Source: CAD feature listing. Evaluate the final solid. Frame: model axes, mm. A direction names the side the tool comes from. Round coordinates to 2 decimals unless told otherwise and drop trailing zeros. Write each loop counter-clockwise with the first axis right and the second up, starting at its lowest first coordinate (ties: lowest second). Pieces come first, ordered by that corner, then holes. Notation, with made-up numbers: (-37, -7.75) -> (-33, -7.75) arc R29 ccw to (-33, 16.25) -> close; hole circle Ø2 at (-35, 73). An arc over 180 degrees is marked (long way). Return JSON: item names as keys, results as strings. Group by question number.
from build123d import *

# Parameters (mm, degrees)
SKETCH2_R           = 13.25
SKETCH2_R_2         = 6
BOSS_EXTRUDE1_DEPTH = 5
SKETCH3_R           = 2.25
SKETCH3_R_2         = 1.25
CUT_EXTRUDE1_DEPTH  = 6


with BuildPart() as part:
    # Sketch2 → Boss-Extrude1 (new body)
    with BuildSketch(Plane.XY):
        with BuildLine():
            ThreePointArc((15.576905983, -13.25), (-20.45, 0), (15.576905983, 13.25))
            Line((15.576905983, 13.25), (25.796075283, 13.25))
            ThreePointArc((25.796075283, 13.25), (-29, 0), (25.796075283, -13.25))
            Line((25.796075283, -13.25), (15.576905983, -13.25))
        make_face()
        with BuildLine():
            ThreePointArc((20.228754287, -3), (18.621948121, -8.451363686), (15.576905983, -13.25))
            Line((15.576905983, -13.25), (25.796075283, -13.25))
            ThreePointArc((25.796075283, -13.25), (27.796785579, -8.266723138), (28.844410204, -3))
            Line((28.844410204, -3), (20.228754287, -3))
        make_face()
        with BuildLine():
            Line((25.796075283, 13.25), (15.576905983, 13.25))
            ThreePointArc((15.576905983, 13.25), (18.621948121, 8.451363686), (20.228754287, 3))
            Line((20.228754287, 3), (28.844410204, 3))
            ThreePointArc((28.844410204, 3), (27.796785579, 8.266723138), (25.796075283, 13.25))
        make_face()
        with BuildLine():
            Line((100, 13.25), (25.796075283, 13.25))
            ThreePointArc((25.796075283, 13.25), (27.796785579, 8.266723138), (28.844410204, 3))
            Line((28.844410204, 3), (50, 3))
            Line((50, 3), (80, 3))
            ThreePointArc((80, 3), (82.121320344, 2.121320344), (83, 0))
            ThreePointArc((83, 0), (82.121320344, -2.121320344), (80, -3))
            Line((80, -3), (50, -3))
            Line((50, -3), (28.844410204, -3))
            ThreePointArc((28.844410204, -3), (27.796785579, -8.266723138), (25.796075283, -13.25))
            Line((25.796075283, -13.25), (100, -13.25))
            ThreePointArc((100, -13.25), (86.75, 0), (100, 13.25))
        make_face()
        with Locations((100, 0)):
            Circle(SKETCH2_R)
        with Locations((100, 0)):
            Circle(SKETCH2_R_2, mode=Mode.SUBTRACT)
    extrude(amount=BOSS_EXTRUDE1_DEPTH)

    # Sketch3 → Cut-Extrude1 (cut, through all)
    with BuildSketch(Plane.XY.offset(5)):
        with Locations((17.67766953, 17.67766953)):
            Circle(SKETCH3_R)
        with Locations((17.67766953, -17.67766953)):
            Circle(SKETCH3_R)
        with Locations((-17.67766953, -17.67766953)):
            Circle(SKETCH3_R)
        with Locations((-17.67766953, 17.67766953)):
            Circle(SKETCH3_R)
        with Locations((100, 10.25)):
            Circle(SKETCH3_R_2)
        with Locations((108.876760389, 5.125)):
            Circle(SKETCH3_R_2)
        with Locations((91.123239611, 5.125)):
            Circle(SKETCH3_R_2)
        with Locations((91.362305232, -5.518399142)):
            Circle(SKETCH3_R_2)
        with Locations((108.876760389, -5.125)):
            Circle(SKETCH3_R_2)
        with Locations((100, -10.25)):
            Circle(SKETCH3_R_2)
    extrude(amount=-CUT_EXTRUDE1_DEPTH, mode=Mode.SUBTRACT)


solid = part.part
Item 1: Pull-direction query (Y, two-part tool) for faces 4 (the cylindrical face through (90.37, -6.28, 2.54)), 5 (the cylindrical face through (113.247, -0.291, 2.465)), 6 (the flat face through (63, 13.25, 2)); classes: +Y half, -Y half, draft (parallel to the pull), parting line (faces both ways), or undercut.
Item 2: Cut plane C-C on z = 0.75. Give the number of separate pieces and of enclosed holes in the cut face, and give its area (3 significant figures).
Item 3: Cut plane D-D on y = -10.25. Output: boundary loops of the cut face in (x, z).
Item 4: First-contact query: pin 1 Ø3 at (y, z) = (-17.5, 1) entering from -X; pin 2 Ø3 at (y, z) = (-19.5, 3.5) entering from -X; pin 3 Ø2.5 at (x, z) = (65, 3) entering from +Y. Flat tips, straight axial feed; report the tip coordinate or a pass-through.
Item 5: Cut plane B-B on x = 61. Output: boundary loops of the cut face in (y, z).
Item 6: Cut plane A-A on x = 0. Output: boundary loops of the cut face in (y, z), and give its area (3 significant figures).
Item 7: Material intervals for probe 1 along Y at (x, z) = (100, 3.6); probe 2 along X at (y, z) = (11, 4.65); probe 3 along X at (y, z) = (-2.5, 3.95), sorted ascending.
Item 8: Set-up query: faces 1 (the flat face through (41, -6, 5)), 2 (the flat face through (62, -13.25, 2)), 3 (the flat face through (50, 3, 2)). Return all of +Z, -Z, +X, -X, +Y, -Y with unobstructed straight access to the full face (end or side cutting, diameter ignored); none if empty.
Here are the results:
{
 "1": {"face 4": "undercut", "face 5": "parting line", "face 6": "+Y half"},
 "2": {"separate pieces": "1", "enclosed holes": "12", "area": "2,940 mm^2"},
 "3": {"outline": "(-27.13, 0) -> (-17.7, 0) -> (-17.7, 5) -> (-27.13, 5) -> close; (17.7, 0) -> (98.75, 0) -> (98.75, 5) -> (17.7, 5) -> close; (101.25, 0) -> (108.4, 0) -> (108.4, 5) -> (101.25, 5) -> close"},
 "4": {"pin 1": "stops at x = -24.19", "pin 2": "stops at x = -22.74", "pin 3": "stops at y = 13.25"},
 "5": {"outline": "(-13.25, 0) -> (-3, 0) -> (-3, 5) -> (-13.25, 5) -> close; (3, 0) -> (13.25, 0) -> (13.25, 5) -> (3, 5) -> close"},
 "6": {"outline": "(-29, 0) -> (-20.45, 0) -> (-20.45, 5) -> (-29, 5) -> close; (20.45, 0) -> (29, 0) -> (29, 5) -> (20.45, 5) -> close", "area": "85.5 mm^2"},
 "7": {"probe 1": "y = -13.25 to -11.5, -9 to -6, 6 to 9, 11.5 to 13.25", "probe 2": "x = -26.83 to -17.24, 17.24 to 99, 101 to 107.39", "probe 3": "x = -28.89 to -20.3, 81.66 to 94.55, 105.45 to 113.01"},
 "8": {"face 1": "+Z, +X, -X, +Y, -Y", "face 2": "+Z, -Z, +X, -Y", "face 3": "+Z, -Z"}
}
